Can you work these out from the model? Positions are in its coordinate system, mm. Give positions to 0.01 mm unless a question says otherwise; leave off trailing zeros. Loops run counter-clockwise (first coordinate to the right, second up) from the corner with the lowest first, then second, coordinate; pieces in that order, holes last. Notation, with made-up numbers: (-20.5, 8) -> (33.5, 8) arc R12 cw to (33.5, 17) -> close; hole circle Ø4 at (72, 22). An arc over 180 degrees is marked (long way). Return JSON: item names as keys, results as strings. Group by question number.
Q1. Thinking about a two-plate mould opening in Z: for faces 1 (the flat face through (-6, -8.188, -64)), 2 (the conical face through (-8, -18, -80)), 3 (the flat face through (-6, -5, -30.97)), 4 (the flat face through (-3.175, -7, -63)), which applies, pulls with the +Z half, pulls with the -Z half, needs draft (parallel to the pull), parting line crosses it, or undercut?
Q2. I need wall thicknesses on line 1 along Y through (x, z) = (-6.45, -46.05); line 2 along Y through (x, z) = (-7.5, -77.5); line 3 along Z through (x, y) = (-4.4, -18.75). Which ranges of each line are inside material? Lowest first, please. Write a range as [from, to].
Q3. Suppose I cut it at A-A, the plane z = -63.5. Count the separate pieces of the cut face and the enclosed holes in it, and give its area (3 significant figures).
Q4. Suppose I cut it at B-B, the plane z = -51.5. Please give me the cut outline in (x, y) (1 decimal).
Q5. Will these pins go through, and if not, where does the flat tip stop? pin 1 (3 mm diameter, centred on y = -19.875, z = -46.05, fed in from +X); pin 2 (4.5 mm diameter, centred on y = -19.875, z = -80.95, fed in from -X); pin 3 (1 mm diameter, centred on x = -7.5, y = -12, fed in from +Z).
```python
from build123d import *

# Parameters (mm, degrees)
SKETCH1_W                = 24
SKETCH1_H                = 65.06
BOSS_EXTRUDE1_DEPTH      = 5
CUT_EXTRUDE1_DEPTH       = 100.109842599
CUT_EXTRUDE2_DEPTH       = 100.109842599
CUT_EXTRUDE3_DEPTH       = 100.109842599
M3_CLEARANCE_HOLE1_D     = 3.556
M3_CLEARANCE_HOLE2_D     = 3.556
F_5_0_5_DIAMETER_HOLE1_D = 5
F_5_0_5_DIAMETER_HOLE2_D = 5
FILLET1_R                = 3
CHAMFER1_SIZE            = 0.5


with BuildPart() as part:
    # Sketch1 → Boss-Extrude1 (new body)
    with BuildSketch(Plane(origin=(-8.175, 0, 0), x_dir=(0, -1, 0), z_dir=(-1, 0, 0))):
        with Locations((12, -63.5)):
            Rectangle(SKETCH1_W, SKETCH1_H)
    extrude(amount=-BOSS_EXTRUDE1_DEPTH)

    # Sketch2 → Cut-Extrude1 (cut, through all)
    with BuildSketch(Plane(origin=(-3.175, 0, 0), x_dir=(0, 0, -1), z_dir=(1, 0, 0))):
        with BuildLine():
            Line((30.97, -24), (45.892842167, -24))
            ThreePointArc((45.892842167, -24), (42.991793175, -23.072335294), (41.167224487, -20.633565899))
            ThreePointArc((41.167224487, -20.633565899), (40.784453665, -19.789293795), (40.252408967, -19.030190819))
            Line((40.252408967, -19.030190819), (30.97, -8.102149698))
            Line((30.97, -8.102149698), (30.97, -24))
        make_face()
    extrude(amount=-CUT_EXTRUDE1_DEPTH, mode=Mode.SUBTRACT)

    # Sketch3 → Cut-Extrude2 (cut, through all)
    with BuildSketch(Plane(origin=(-3.175, 0, 0), x_dir=(0, 0, -1), z_dir=(1, 0, 0))):
        with BuildLine():
            Line((81.4047462, -24), (96.03, -24))
            Line((96.03, -24), (96.03, -8.102149698))
            Line((96.03, -8.102149698), (87.219197841, -18.474975184))
            ThreePointArc((87.219197841, -18.474975184), (86.616905128, -19.361470748), (86.2173731, -20.355958082))
            ThreePointArc((86.2173731, -20.355958082), (84.423041214, -22.986213141), (81.4047462, -24))
        make_face()
    extrude(amount=-CUT_EXTRUDE2_DEPTH, mode=Mode.SUBTRACT)

    # Sketch4 → Cut-Extrude3 (cut, through all)
    with BuildSketch(Plane(origin=(-3.175, 0, 0), x_dir=(0, 0, -1), z_dir=(1, 0, 0))):
        with BuildLine():
            Line((80.95, -8.1875), (46.05, -8.1875))
            ThreePointArc((46.05, -8.1875), (42.3, -11.9375), (46.05, -15.6875))
            Line((46.05, -15.6875), (80.95, -15.6875))
            ThreePointArc((80.95, -15.6875), (84.7, -11.9375), (80.95, -8.1875))
        make_face()
    extrude(amount=-CUT_EXTRUDE3_DEPTH, mode=Mode.SUBTRACT)

    # M3 Clearance Hole1 (through all)
    with Locations(Plane.ZY.offset(8.175)):
        with Locations((-46.05, -4)):
            Hole(M3_CLEARANCE_HOLE1_D / 2)

    # M3 Clearance Hole2 (through all)
    with Locations(Plane(origin=(-3.175, 0, 0), x_dir=(0, 0, -1), z_dir=(1, 0, 0))):
        with Locations((46.05, -19.875), (63.5, -19.875), (80.95, -19.875), (80.95, -4), (63.5, -4)):
            Hole(M3_CLEARANCE_HOLE2_D / 2)

    # Ø5.0 (5) Diameter Hole1 (through all)
    with Locations(Plane.ZY.offset(8.175)):
        with Locations((-91.03, -5)):
            Hole(F_5_0_5_DIAMETER_HOLE1_D / 2)

    # Ø5.0 (5) Diameter Hole2 (through all)
    with Locations(Plane(origin=(-3.175, 0, 0), x_dir=(0, 0, -1), z_dir=(1, 0, 0))):
        with Locations((35.97, -5)):
            Hole(F_5_0_5_DIAMETER_HOLE2_D / 2)

    # Fillet1
    fillet1_edges = [part.edges().sort_by_distance(p)[0] for p in [
        (-5.675, -8.102149698, -30.97),
        (-5.675, -8.102149698, -96.03),
        (-5.675, 0, -96.03),
        (-5.675, 0, -30.97),
    ]]
    fillet(fillet1_edges, radius=FILLET1_R)

    # Chamfer1
    chamfer1_edges = [part.edges().sort_by_distance(p)[0] for p in [
        (-8.175, -5, -88.53),
        (-3.175, -5, -88.53),
        (-3.175, -5, -38.47),
        (-8.175, -5, -38.47),
        (-8.175, -5, -30.97),
        (-3.175, -5, -30.97),
        (-3.175, -13.708569886, -91.267839568),
        (-3.175, -5, -96.03),
        (-3.175, 0, -63.5),
        (-3.175, -8.034542438, -95.845976197),
        (-3.175, -0.878679656, -31.848679656),
        (-3.175, -0.878679656, -95.151320344),
        (-3.175, -8.034542438, -31.154023803),
        (-8.175, -5, -96.03),
        (-8.175, -13.708569886, -91.267839568),
        (-8.175, 0, -63.5),
        (-8.175, -8.034542438, -95.845976197),
        (-8.175, -0.878679656, -31.848679656),
        (-8.175, -0.878679656, -95.151320344),
        (-8.175, -8.034542438, -31.154023803),
        (-8.175, -13.986177703, -35.967963836),
        (-8.175, -19.789293795, -40.784453665),
        (-8.175, -23.072335294, -42.991793175),
        (-3.175, -23.072335294, -42.991793175),
        (-3.175, -19.789293795, -40.784453665),
        (-3.175, -13.986177703, -35.967963836),
        (-8.175, -24, -63.648794183),
        (-3.175, -24, -63.648794183),
        (-8.175, -19.361470748, -86.616905128),
        (-8.175, -22.986213141, -84.423041214),
        (-3.175, -19.361470748, -86.616905128),
        (-3.175, -22.986213141, -84.423041214),
        (-8.175, -11.9375, -84.7),
        (-8.175, -15.6875, -63.5),
        (-8.175, -11.9375, -42.3),
        (-8.175, -8.1875, -63.5),
        (-3.175, -11.9375, -84.7),
        (-3.175, -8.1875, -63.5),
        (-3.175, -11.9375, -42.3),
        (-3.175, -15.6875, -63.5),
        (-8.175, -4, -44.272),
        (-3.175, -4, -44.272),
        (-3.175, -4, -65.278),
        (-8.175, -4, -65.278),
        (-3.175, -4, -82.728),
        (-8.175, -4, -82.728),
        (-3.175, -19.875, -82.728),
        (-8.175, -19.875, -82.728),
        (-3.175, -19.875, -65.278),
        (-8.175, -19.875, -65.278),
        (-3.175, -19.875, -47.828),
        (-8.175, -19.875, -47.828),
    ]]
    chamfer(chamfer1_edges, length=CHAMFER1_SIZE)


solid = part.part
```
Ans:
{
 "1": {"face 1": "undercut", "face 2": "undercut", "face 3": "pulls with the +Z half", "face 4": "needs draft"},
 "2": {"line 1": "y = [-24, -21.65], [-18.1, -15.69], [-8.19, -5.78], [-2.22, 0]", "line 2": "y = [-24, -15.69], [-8.19, 0]", "line 3": "z = [-87, -82.33], [-79.57, -64.88], [-62.12, -47.43], [-44.67, -40.01]"},
 "3": {"separate pieces": "4", "enclosed holes": "0", "area": "44.9 mm^2"},
 "4": {"outline": "(-8.2, -23.5) -> (-7.7, -24) -> (-3.7, -24) -> (-3.2, -23.5) -> (-3.2, -16.2) -> (-3.7, -15.7) -> (-7.7, -15.7) -> (-8.2, -16.2) -> close; (-8.2, -7.7) -> (-7.7, -8.2) -> (-3.7, -8.2) -> (-3.2, -7.7) -> (-3.2, -0.5) -> (-3.7, 0) -> (-7.7, 0) -> (-8.2, -0.5) -> close"},
 "5": {"pin 1": "passes through", "pin 2": "stops at x = -8.15", "pin 3": "stops at z = -33.86"}
}
